Geometry: final body of the model. Coordinates: model frame, mm. A direction names the side the tool comes from. Round coordinates to 2 decimals unless told otherwise and drop trailing zeros. Order: outer loops, then holes, each group sorted by start corner. A loop starts at its lowest first (then second) coordinate and runs counter-clockwise, first axis right, second up. Notation, with made-up numbers: (70.5, 48.5) -> (126.5, 48.5) arc R24 cw to (126.5, 80.5) -> close; hole circle Ø11 at (-33, 78). An arc over 180 degrees is marked (long way). Put each result on its own line as item: value.
```python
from build123d import *

# Parameters (mm, degrees)
BOSS_EXTRUDE1_DEPTH = 2
SKETCH2_W           = 5
SKETCH2_H           = 1.5
BOSS_EXTRUDE2_DEPTH = 1
SKETCH3_W           = 1.5
SKETCH3_H           = 11
BOSS_EXTRUDE4_DEPTH = 1
SKETCH4_R           = 1
CUT_EXTRUDE1_DEPTH  = 47.184412955
LPATTERN1_COUNT     = 2
LPATTERN1_PITCH     = 6


with BuildPart() as part:
    # Sketch1 → Boss-Extrude1 (new body)
    with BuildSketch(Plane(origin=(0, 0, 0), x_dir=(1, 0, 0), z_dir=(0, 1, 0))):
        Polygon((5.25, -40), (5.25, -30), (0, -30), (0, 0), (23, 0), (23, -30), (17.75, -30), (17.75, -40), align=None)
    extrude(amount=BOSS_EXTRUDE1_DEPTH)

    # Sketch2 → Boss-Extrude2 (add)
    with BuildSketch(Plane(origin=(0, 2, 0), x_dir=(1, 0, 0), z_dir=(0, 1, 0))):
        Polygon((3.88999026, -13.440542412), (5.38999026, -13.440542412), (5.38999026, -15.690542412), (6.88999026, -15.690542412), (6.88999026, -9.690542412), (5.38999026, -9.690542412), (5.38999026, -11.940542412), (3.88999026, -11.940542412), (2.38999026, -11.940542412), (2.38999026, -13.440542412), (2.38999026, -28.962116838), (3.88999026, -28.962116838), align=None)
        with Locations((8.38999026, -7.940542412)):
            Rectangle(SKETCH2_W, SKETCH2_H)
        with Locations((8.38999026, -17.440542412)):
            Rectangle(SKETCH2_W, SKETCH2_H)
        Polygon((11.38999026, -9.690542412), (9.88999026, -9.690542412), (9.88999026, -15.690542412), (11.38999026, -15.690542412), (11.38999026, -13.440542412), (12.88999026, -13.440542412), (12.88999026, -28.962116838), (14.38999026, -28.962116838), (14.38999026, -13.440542412), (14.38999026, -11.940542412), (12.88999026, -11.940542412), (11.38999026, -11.940542412), align=None)
    extrude(amount=BOSS_EXTRUDE2_DEPTH)

    # Sketch3 → Boss-Extrude4 (add)
    with BuildSketch(Plane(origin=(0, 2, 0), x_dir=(1, 0, 0), z_dir=(0, 1, 0))):
        with Locations((8.38999026, -23.690542412)):
            Rectangle(SKETCH3_W, SKETCH3_H)
        Polygon((7.63999026, -4.190542412), (7.63999026, -7.190542412), (9.13999026, -7.190542412), (9.13999026, -5.690542412), (17.646471735, -5.690542412), (17.646471735, -28.690542412), (19.146471735, -28.690542412), (19.146471735, -4.190542412), align=None)
    extrude(amount=BOSS_EXTRUDE4_DEPTH)

    # Sketch4 → Cut-Extrude1 (cut, through all)
    with BuildSketch(Plane(origin=(0, 2, 0), x_dir=(1, 0, 0), z_dir=(0, 1, 0))):
        with Locations(Location((11.5, -37.5, 0), (0, 0, 270))):
            Circle(SKETCH4_R)
    cut_extrude1 = extrude(amount=-CUT_EXTRUDE1_DEPTH, mode=Mode.SUBTRACT)

    # LPattern1: Cut-Extrude1 ×2
    with Locations(*[(0, 0, -i * LPATTERN1_PITCH) for i in range(1, LPATTERN1_COUNT)]):
        add(cut_extrude1, mode=Mode.SUBTRACT)


solid = part.part
```
1. Cut plane D-D on z = 35.5. Return loops of the section in (x, y), and give its area (3 significant figures).
Ans:
outline: (5.25, 0) -> (17.75, 0) -> (17.75, 2) -> (5.25, 2) -> close
area: 25.0 mm²
2. Cut plane A-A on z = 31.5. Return loops of the section in (x, y), and give its area (3 significant figures).
Ans:
outline: (5.25, 0) -> (10.5, 0) -> (10.5, 2) -> (5.25, 2) -> close; (12.5, 0) -> (17.75, 0) -> (17.75, 2) -> (12.5, 2) -> close
area: 21.0 mm²
3. Contact query for flat-ended pins moving along their axis: P1, Ø0.5, axis at y = 2.5, z = 14, coming from the +X side; P2, Ø0.5, axis at x = 4, y = 2.5, coming from the -Z side; P3, Ø0.5, axis at y = 2.5, z = 5, coming from the -X side; P4, Ø1.5, axis at y = 2.5, z = 18, coming from the +X side. Output: stop coordinate, or through.
Ans:
P1: x = 19.15
P2: z = 11.94
P3: x = 7.64
P4: x = 23
4. Cut plane C-C on x = 1.75. Return loops of the section in (y, z).
Ans:
outline: (0, 0) -> (2, 0) -> (2, 30) -> (0, 30) -> close
5. Set-up query: faces 5 (the face through (3, 1, 30)), 6 (the face through (8.4, 2.5, 8.691)), 7 (the face through (2.39, 2.5, 20.3)), 8 (the face through (10.89, 2.5, 8)). Return all of +Z, -Z, +X, -X, +Y, -Y with unobstructed straight access to the full face (end or side cutting, diameter ignored); none if empty.
Ans:
face 5: +Z, -X, +Y, -Y
face 6: -X, +Y
face 7: +Z, -Z, -X, +Y
face 8: +Y
6. Draft query along Z for faces 1 (the face through (19.146, 2.5, 16.6)), 2 (the face through (11, 1, 0)), 3 (the face through (10.524, 1.014, 31.283)), 4 (the face through (10, 2.5, 18.191)). Return one class per face: +Z half, -Z half, draft (parallel to the pull), parting line (faces both ways), or undercut.
Ans:
face 1: draft
face 2: -Z half
face 3: undercut
face 4: +Z half
7. Material intervals for probe 1 along Z at (x, y) = (9.5, 2.05); probe 2 along Z at (x, y) = (12, 2.6); probe 3 along X at (y, z) = (0.4, 37.5), sorted ascending.
Ans:
probe 1: 4.19 to 5.69, 7.19 to 8.69, 16.69 to 18.19
probe 2: 4.19 to 5.69, 11.94 to 13.44
probe 3: 5.25 to 10.5, 12.5 to 17.75
8. Cut plane B-B on y = 1.4. Return loops of the section in (x, z).
Ans:
outline: (0, 0) -> (23, 0) -> (23, 30) -> (17.75, 30) -> (17.75, 40) -> (5.25, 40) -> (5.25, 30) -> (0, 30) -> close; hole circle Ø2 at (11.5, 31.5); hole circle Ø2 at (11.5, 37.5)
